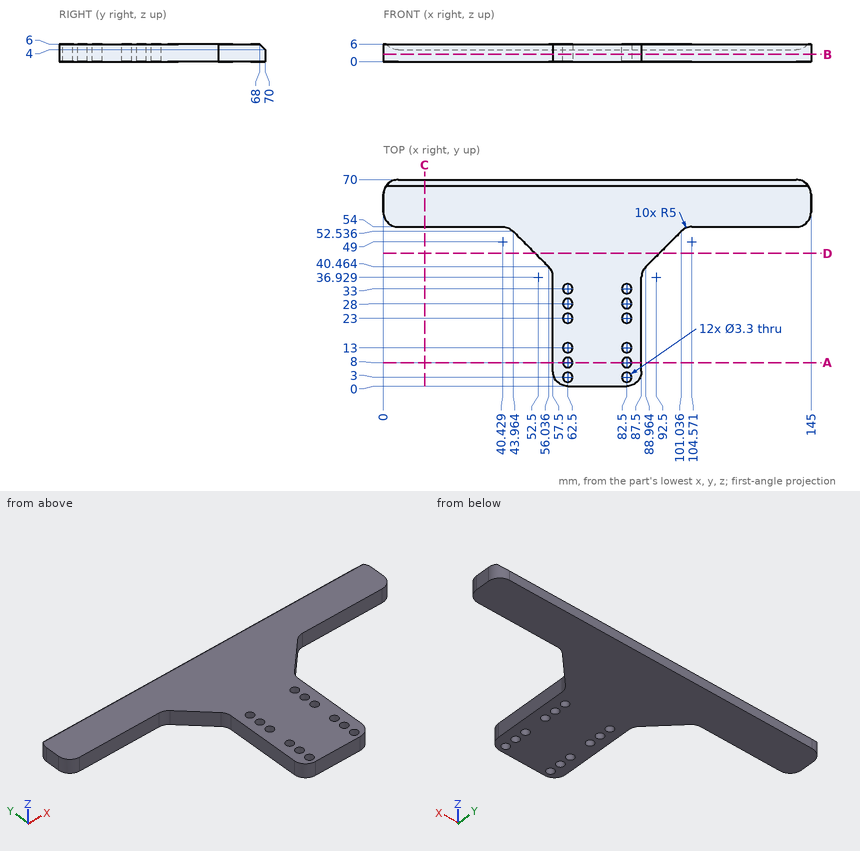
Answer from the drawing. Dimensions are ordinates in mm from the lowest x, y and z of the part. Give positions to 0.01 mm unless a question says otherwise; leave off trailing zeros. Loops run counter-clockwise (first coordinate to the right, second up) from the corner with the lowest first, then second, coordinate; pieces in that order, holes last.
Item 1: Find the intervals of material crossed by line 1 along Y through (x, z) = (26, 1); line 2 along X through (y, z) = (5, 1.25); line 3 along Y through (x, z) = (52, 3.5), in increasing order.
Derived:
line 1: y = 54 to 70
line 2: x = 57.5 to 87.5
line 3: y = 44.5 to 70
Item 2: A cutting plane is placed at D-D (y = 45). Give the vertices of the cut face in (x, z), then the cut area to 3 significant figures.
Derived:
outline: (51.5, 0) - (93.5, 0) - (93.5, 6) - (51.5, 6) - close
area: 252 mm2
Item 3: A cutting plane is placed at C-C (x = 14). Give the vertices of the cut face in (y, z).
Derived:
outline: (54, 0) - (70, 0) - (70, 4) - (68, 6) - (54, 6) - close
Item 4: A cutting plane is placed at A-A (y = 8). Give the vertices of the cut face in (x, z).
Derived:
outline: (57.5, 0) - (60.85, 0) - (60.85, 6) - (57.5, 6) - close; (64.15, 0) - (80.85, 0) - (80.85, 6) - (64.15, 6) - close; (84.15, 0) - (87.5, 0) - (87.5, 6) - (84.15, 6) - close
Item 5: A cutting plane is placed at B-B (z = 2.5). Give the number of separate pieces and of enclosed holes in the cut face, then the cut area to 3 significant figures.
Derived:
separate pieces: 1
enclosed holes: 12
area: 4,030 mm2
Item 6: Each of these flat-tipped pins is pushed along its axis until it touches: pin 1 Ø2 at (y, z) = (45.5, 3) entering from -X; pin 2 Ø1 at (y, z) = (24, 3.5) entering from -X; pin 3 Ø1.5 at (x, z) = (23.5, 1) entering from -Y. Where does it stop, or does it pass through?
Derived:
pin 1: stops at x = 50
pin 2: stops at x = 57.5
pin 3: stops at y = 54
